Source: three-view drawing plus pictorial views. Frame: mm from the lowest corner of the part. Coordinates: 2 decimals unless noted, no trailing zeros. Order: outer loops, then holes, each group sorted by start corner. A loop starts at its lowest first (then second) coordinate and runs counter-clockwise, first axis right, second up. Notation, with made-up numbers: M 0.25,-28.5 L 12.25,-28.5 A28 ccw 12.25,6.5 Z; hole C 79.25,14.25 d10. An arc over 180 degrees is marked long. Write item = value, one per line. Start each with the question number.
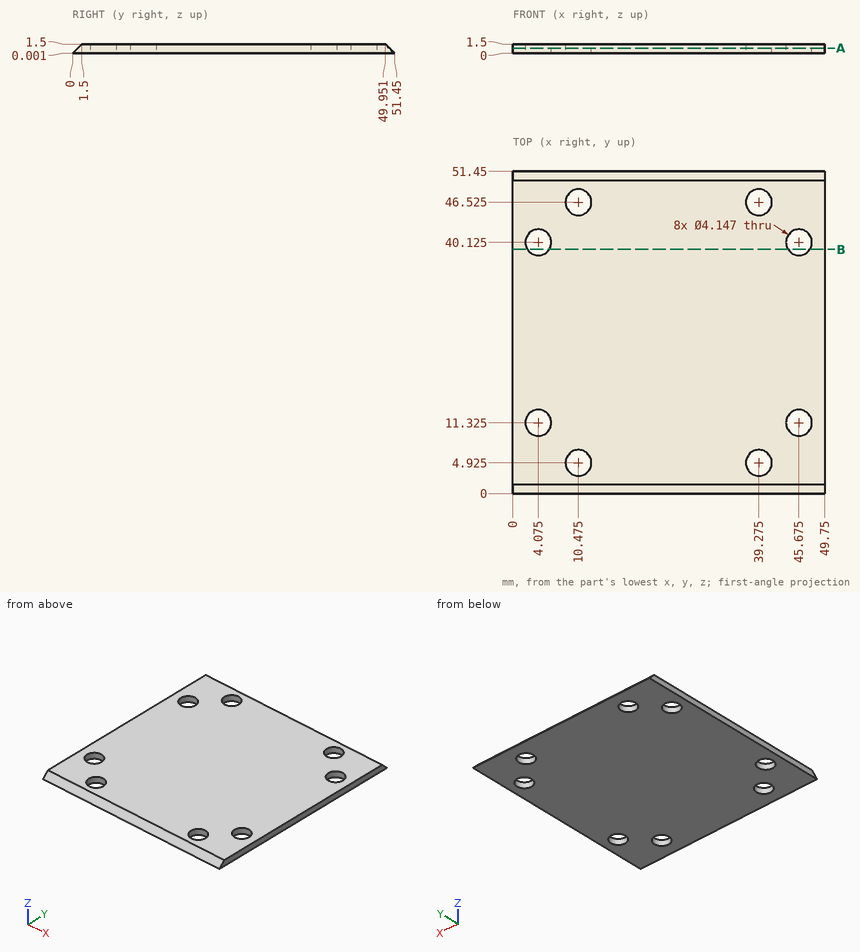
Item 1: Material intervals for probe 1 along Y at (x, z) = (12, 0.5); probe 2 along Y at (x, z) = (45.5, 0.2); probe 3 along Y at (x, z) = (48, 0.2), sorted ascending. Write a range as [from, to].
Item 2: Section query B-B on y = 39. Output: boundary loops of the cut face in (x, z).
Item 3: Section query A-A on z = 0.85. Give the number of separate pieces and of enclosed holes in the cut face, and give its area (3 significant figures).
Ans:
q1.probe_1 = [0.5, 3.52], [6.33, 45.12], [47.93, 50.95]
q1.probe_2 = [0.2, 9.26], [13.39, 38.06], [42.19, 51.25]
q1.probe_3 = [0.2, 51.25]
q2.outline = M 0,0 L 2.33,0 L 2.33,1.5 L 0,1.5 Z; M 5.82,0 L 43.93,0 L 43.93,1.5 L 5.82,1.5 Z; M 47.42,0 L 49.75,0 L 49.75,1.5 L 47.42,1.5 Z
q3.separate_pieces = 1
q3.enclosed_holes = 8
q3.area = 2,370 mm^2
